The listing builds one solid part. Answer for the finished solid, in the listing's coordinates (mm). Give positions to 0.01 mm unless a question says otherwise; leave off trailing zeros. Order: outer loops, then holes, each group sorted by start corner. A loop starts at its lowest first (then second) coordinate and runs counter-clockwise, first axis right, second up. Notation, with made-up numbers: (67, 40) - (71, 40) arc R23 cw to (71, 76) - close; hole circle Ø3 at (-26, 30). An arc over 180 degrees is marked (long way). Answer in a Markdown table with one row per item.
from build123d import *

# Parameters (mm, degrees)
SKETCH1_W           = 31.75
SKETCH1_H           = 25.4
BOSS_EXTRUDE1_DEPTH = 1.524
CUT_EXTRUDE1_REACH  = 22.387
SKETCH2_R           = 1.9812
CUT_EXTRUDE2_REACH  = 22.387
SKETCH3_R           = 0.75
LPATTERN1_COUNT     = 5
LPATTERN1_PITCH     = 2.54
CUT_EXTRUDE3_REACH  = 22.387
SKETCH4_R           = 0.7493


with BuildPart() as part:
    # Sketch1 → Boss-Extrude1 (new body)
    with BuildSketch(Plane(origin=(0, 0, 0), x_dir=(1, 0, 0), z_dir=(0, 1, 0))):
        Rectangle(SKETCH1_W, SKETCH1_H)
    extrude(amount=BOSS_EXTRUDE1_DEPTH)

    # Sketch2 → Cut-Extrude1 (cut, up to next)
    with BuildSketch(Plane(origin=(0, 1.524, 0), x_dir=(1, 0, 0), z_dir=(0, 1, 0)), mode=Mode.PRIVATE) as cut_extrude1_sk1:
        with Locations(Location((-13.335, 10.16, 0), (0, 0, 270))):
            Circle(SKETCH2_R)
    cut_extrude1_tool1 = extrude(cut_extrude1_sk1.sketch, amount=-CUT_EXTRUDE1_REACH, mode=Mode.PRIVATE) & part.part
    # Sketch2 → Cut-Extrude1 (cut, up to next)
    with BuildSketch(Plane(origin=(0, 1.524, 0), x_dir=(1, 0, 0), z_dir=(0, 1, 0)), mode=Mode.PRIVATE) as cut_extrude1_sk2:
        with Locations(Location((13.335, 10.16, 0), (0, 0, 90))):
            Circle(SKETCH2_R)
    cut_extrude1_tool2 = extrude(cut_extrude1_sk2.sketch, amount=-CUT_EXTRUDE1_REACH, mode=Mode.PRIVATE) & part.part
    # Sketch2 → Cut-Extrude1 (cut, up to next)
    with BuildSketch(Plane(origin=(0, 1.524, 0), x_dir=(1, 0, 0), z_dir=(0, 1, 0)), mode=Mode.PRIVATE) as cut_extrude1_sk3:
        with Locations(Location((-13.335, -10.16, 0), (0, 0, 90))):
            Circle(SKETCH2_R)
    cut_extrude1_tool3 = extrude(cut_extrude1_sk3.sketch, amount=-CUT_EXTRUDE1_REACH, mode=Mode.PRIVATE) & part.part
    # Sketch2 → Cut-Extrude1 (cut, up to next)
    with BuildSketch(Plane(origin=(0, 1.524, 0), x_dir=(1, 0, 0), z_dir=(0, 1, 0)), mode=Mode.PRIVATE) as cut_extrude1_sk4:
        with Locations(Location((13.335, -10.16, 0), (0, 0, 270))):
            Circle(SKETCH2_R)
    cut_extrude1_tool4 = extrude(cut_extrude1_sk4.sketch, amount=-CUT_EXTRUDE1_REACH, mode=Mode.PRIVATE) & part.part
    add(cut_extrude1_tool1.solids().sort_by_distance((-13.335, 1.524, -10.16))[0], mode=Mode.SUBTRACT)
    add(cut_extrude1_tool2.solids().sort_by_distance((13.335, 1.524, -10.16))[0], mode=Mode.SUBTRACT)
    add(cut_extrude1_tool3.solids().sort_by_distance((-13.335, 1.524, 10.16))[0], mode=Mode.SUBTRACT)
    add(cut_extrude1_tool4.solids().sort_by_distance((13.335, 1.524, 10.16))[0], mode=Mode.SUBTRACT)

    # Sketch3 → Cut-Extrude2 (cut, up to next)
    with BuildSketch(Plane(origin=(0, 1.524, 0), x_dir=(1, 0, 0), z_dir=(0, 1, 0)), mode=Mode.PRIVATE) as cut_extrude2_sk1:
        with Locations(Location((-14.605, 5.08, 0), (0, 0, 270))):
            Circle(SKETCH3_R)
    cut_extrude2_tool1 = extrude(cut_extrude2_sk1.sketch, amount=-CUT_EXTRUDE2_REACH, mode=Mode.PRIVATE) & part.part
    cut_extrude2 = cut_extrude2_tool1.solids().sort_by_distance((-14.605, 1.524, -5.08))[0]
    add(cut_extrude2, mode=Mode.SUBTRACT)

    # LPattern1: Cut-Extrude2 ×5
    with Locations(*[(0, 0, i * LPATTERN1_PITCH) for i in range(1, LPATTERN1_COUNT)]):
        add(cut_extrude2, mode=Mode.SUBTRACT)

    # Sketch4 → Cut-Extrude3 (cut, up to next)
    with BuildSketch(Plane(origin=(0, 1.524, 0), x_dir=(1, 0, 0), z_dir=(0, 1, 0)), mode=Mode.PRIVATE) as cut_extrude3_sk1:
        with Locations(Location((1.8288, 0.0762, 0), (0, 0, 270))):
            Circle(SKETCH4_R)
    cut_extrude3_tool1 = extrude(cut_extrude3_sk1.sketch, amount=-CUT_EXTRUDE3_REACH, mode=Mode.PRIVATE) & part.part
    add(cut_extrude3_tool1.solids().sort_by_distance((1.8288, 1.524, -0.0762))[0], mode=Mode.SUBTRACT)


solid = part.part
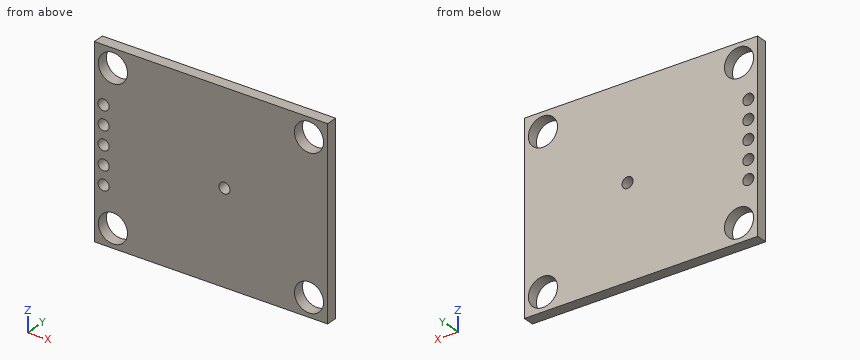
Item 1: Find section D-D on z = -10.5. Write down the section's boundary in (x, y) (3 decimals).
Answer block:
| item | result |
|---|---|
| outline | (-15.875, 0) - (-15.287, 0) - (-15.287, 1.524) - (-15.875, 1.524) - close; (-11.383, 0) - (11.383, 0) - (11.383, 1.524) - (-11.383, 1.524) - close; (15.287, 0) - (15.875, 0) - (15.875, 1.524) - (15.287, 1.524) - close |
Item 2: Find section C-C on y = 0.45. Count the separate pieces of the cut face and the enclosed holes in it, then the cut area to 3 significant figures.
Answer block:
| item | result |
|---|---|
| separate pieces | 1 |
| enclosed holes | 10 |
| area | 747 mm² |
Item 3: Find section B-B on z = 10.16. Write down the section's boundary in (x, y) (3 decimals), then the cut area to 3 significant figures.
Answer block:
| item | result |
|---|---|
| outline | (-15.875, 0) - (-15.316, 0) - (-15.316, 1.524) - (-15.875, 1.524) - close; (-11.354, 0) - (11.354, 0) - (11.354, 1.524) - (-11.354, 1.524) - close; (15.316, 0) - (15.875, 0) - (15.875, 1.524) - (15.316, 1.524) - close |
| area | 36.3 mm² |
Item 4: Consider line 1 (X direction, y = 0.75, z = 10.16) (3 decimals); line 2 (X direction, y = 0.4, z = 0) (3 decimals); line 3 (X direction, y = 0.8, z = 2.54) (3 decimals). Determine where each line is inside the solid, lowest interval first.
Answer block:
| item | result |
|---|---|
| line 1 | -15.875 to -15.316, -11.354 to 11.354, 15.316 to 15.875 |
| line 2 | -15.875 to -15.355, -13.855 to 1.083, 2.574 to 15.875 |
| line 3 | -15.875 to -15.355, -13.855 to 15.875 |
Item 5: Find section A-A on z = -2.54. Write down the section's boundary in (x, y) (3 decimals), then the cut area to 3 significant figures.
Answer block:
| item | result |
|---|---|
| outline | (-15.875, 0) - (-15.355, 0) - (-15.355, 1.524) - (-15.875, 1.524) - close; (-13.855, 0) - (15.875, 0) - (15.875, 1.524) - (-13.855, 1.524) - close |
| area | 46.1 mm² |
